Verification items for the finished model (mm, model axes). A direction names the side the tool comes from. Round coordinates to 2 decimals unless told otherwise and drop trailing zeros. Loops run counter-clockwise (first coordinate to the right, second up) from the corner with the lowest first, then second, coordinate; pieces in that order, holes last.
from build123d import *

# Parameters (mm, degrees)
SKETCH1_W           = 5
SKETCH1_H           = 190
SKETCH1_H_2         = 5
BOSS_EXTRUDE1_DEPTH = 150
BOSS_EXTRUDE2_DEPTH = 5


with BuildPart() as part:
    # Sketch1 → Boss-Extrude1 (new, symmetric)
    with BuildSketch(Plane(origin=(0, 0, 0), x_dir=(0, 0, -1), z_dir=(1, 0, 0))):
        with Locations((0, 95)):
            Rectangle(SKETCH1_W, SKETCH1_H)
        with Locations((-5, 187.5)):
            Rectangle(SKETCH1_W, SKETCH1_H_2)
        with Locations((5, 2.5)):
            Rectangle(SKETCH1_W, SKETCH1_H_2)
        with Locations((-5, 2.5)):
            Rectangle(SKETCH1_W, SKETCH1_H_2)
    extrude(amount=BOSS_EXTRUDE1_DEPTH, both=True)

    # Sketch2 → Boss-Extrude2 (add)
    with BuildSketch(Plane(origin=(0, 190, 0), x_dir=(1, 0, 0), z_dir=(0, 1, 0))):
        Polygon((135, -7.5), (135, -21.5), (120, -21.5), (120, -16.5), (130, -16.5), (130, -7.5), align=None)
        Polygon((0, -7.5), (5, -7.5), (5, -21.5), (-10, -21.5), (-10, -16.5), (0, -16.5), align=None)
        Polygon((-130, -7.5), (-125, -7.5), (-125, -21.5), (-140, -21.5), (-140, -16.5), (-130, -16.5), align=None)
    extrude(amount=-BOSS_EXTRUDE2_DEPTH)


solid = part.part
1. Release check for a two-part mould opening along Y. For faces 1 (the face through (2, 0, 0)), 2 (the face through (2, 96, -2.5)), 3 (the face through (2, 94, 2.5)), 4 (the face through (2, 190, 4)) record: released by +Y, released by -Y, zero draft, split by the parting line, or undercut.
2. Gauge pin test, flat ends, axial feed: P1, Ø4, axis at y = 188, z = 12, coming from the -X side; P2, Ø10, axis at x = 25.5, y = 107, coming from the +Z side; P3, Ø6, axis at x = -8, z = -1, coming from the -Y side; P4, Ø4, axis at y = 187.5, z = 19, coming from the -X side. Record the tip position at first contact, or that the pin passes through.
3. Section check C-C (y = 32.5). Enter the section's corners in (x, z).
4. Tool access check on faces 5 (the face through (150, 88, 1)), 6 (the face through (1, 185, 7)). Record the directions out of +Z, -Z, +X, -X, +Y, -Y that give a thin tool (end or side, any length) a straight path to the whole face; none if there is none.
5. Section check B-B (x = -78.5). Enter the section's corners in (y, z), then the cut area to 4 significant figures.
6. Section check A-A (z = 11). Enter the section's corners in (x, y).
7. Scan lines: L1, parallel to Y at x = 121, z = 5; L2, parallel to Z at x = 84.5, y = 19.5; L3, parallel to Y at x = 118, z = -6.5. Record each from-to range of solid material in increasing order.
Taken from the geometry:
1. face 1: released by -Y
1. face 2: zero draft
1. face 3: undercut
1. face 4: released by +Y
2. P1: stops at x = -130
2. P2: stops at z = 2.5
2. P3: stops at y = 0
2. P4: stops at x = -140
3. outline: (-150, -2.5) - (150, -2.5) - (150, 2.5) - (-150, 2.5) - close
4. face 5: +Z, -Z, +X, +Y, -Y
4. face 6: +Z, +X, -X
5. outline: (0, -7.5) - (5, -7.5) - (5, -2.5) - (190, -2.5) - (190, 7.5) - (185, 7.5) - (185, 2.5) - (5, 2.5) - (5, 7.5) - (0, 7.5) - close
5. area: 1,025 mm2
6. outline: (-130, 185) - (-125, 185) - (-125, 190) - (-130, 190) - close; (0, 185) - (5, 185) - (5, 190) - (0, 190) - close; (130, 185) - (135, 185) - (135, 190) - (130, 190) - close
7. L1: y = 0 to 5, 185 to 190
7. L2: z = -2.5 to 2.5
7. L3: y = 0 to 5
